```python
from build123d import *

# Parameters (mm, degrees)
F0_W     = 5
F0_H     = 5
F1_DEPTH = 33
F2_R     = 5
F3_DEPTH = 5
F5_DEPTH = 1
F7_W     = 5
F7_H     = 5
F8_DEPTH = 8


with BuildPart() as f1:
    # F0 (on Right) → F1 (new body)
    with BuildSketch(Plane.YZ):
        Rectangle(F0_W, F0_H)
    extrude(amount=F1_DEPTH)

    # F2 (on face) → F3 (join)
    with BuildSketch(Plane.YZ.offset(33)):
        Circle(F2_R)
    extrude(amount=F3_DEPTH)

    # F4 (on face) → F5 (join)
    with BuildSketch(Plane(origin=(0, 0, 0), x_dir=(0, -1, 0), z_dir=(-1, 0, 0))):
        with BuildLine():
            ThreePointArc((0, -2.5), (1.767767, -1.767767), (2.5, 0))
            ThreePointArc((2.5, 0), (1.767767, 1.767767), (0, 2.5))
            ThreePointArc((0, 2.5), (-1.767767, 1.767767), (-2.5, 0))
            ThreePointArc((-2.5, 0), (-1.767767, -1.767767), (0, -2.5))
        make_face()
    extrude(amount=F5_DEPTH)

    # F7 (on face) → F8 (join)
    with BuildSketch(Plane(origin=(-1, 0, 0), x_dir=(0, -1, 0), z_dir=(-1, 0, 0))):
        with Locations((-0.012615, 0.104109)):
            Rectangle(F7_W, F7_H)
    extrude(amount=F8_DEPTH)


solid = f1.part
```
The model under review builds one solid part; all positions refer to its coordinate system, in mm. A direction names the side the tool comes from. Coordinates: 2 decimals unless noted, no trailing zeros. Order: outer loops, then holes, each group sorted by start corner. A loop starts at its lowest first (then second) coordinate and runs counter-clockwise, first axis right, second up. Notation, with made-up numbers: (-1.5, -34.5) -> (51.5, -34.5) arc R17 ccw to (51.5, -8.5) -> close; hole circle Ø1 at (-2.5, -26.75). An arc over 180 degrees is marked (long way). Answer in a Markdown table with one row per item. Add a question column.
Item 1: Mouldability with a two-part tool opening along X and no side actions: class faces 6 (the flat face through (-9, 0, 0)), 7 (the flat face through (-1, 1.32, 2.34)), 8 (the flat face through (16, 0, -2.5)) as +X half, -X half, draft (parallel to the pull), parting line (faces both ways), or undercut.
Item 2: Clearance check with flat-ended pins moving along their axes: pin 1 (6 mm diameter, centred on x = 25.5, y = -3, fed in from +Z); pin 2 (4 mm diameter, centred on x = 12.5, y = 2, fed in from -Z); pin 3 (2.5 mm diameter, centred on x = 23, z = -1, fed in from -Y). State where each tip first meets the part, or that it passes through.
Item 3: We need section A-A on z = 1.75. Write out the cut boundary in (x, y), plus the area to 3 significant figures.
Item 4: We need section B-B on x = -6. Write out the cut boundary in (y, z).
Item 5: We need section C-C on y = -4.5. Write out the cut boundary in (x, z), plus the area to 3 significant figures.
Item 6: We need section D-D on z = -2. Write out the cut boundary in (x, y).
Item 7: Machinability: for faces 1 (the flat face through (0, 2, -2)), 2 (the flat face through (-5, -2.487, 0)), 3 (the flat face through (0, 2, 2)), 4 (the flat face through (0, -2, 2)), 5 (the flat face through (-5, 0, 2.604)), which of the approach directions +Z, -Z, +X, -X, +Y, -Y give a long, thin tool a straight path to every point of the face, cutting with its end or side? Answer none if there is none.
Item 8: To check wall thickness, follow probe 1 along X at (y, z) = (3.25, 2.75); probe 2 along Z at (x, y) = (22.5, 1). State the ranges of each line that lie inside material, in increasing order.
Final values:
| question | item | result |
|---|---|---|
| 1 | face 6 | -X half |
| 1 | face 7 | undercut |
| 1 | face 8 | draft |
| 2 | pin 1 | stops at z = 2.5 |
| 2 | pin 2 | stops at z = -2.5 |
| 2 | pin 3 | stops at y = -2.5 |
| 3 | outline | (-9, -2.49) -> (-1, -2.49) -> (-1, -1.79) -> (0, -1.79) -> (0, -2.5) -> (33, -2.5) -> (33, -4.68) -> (38, -4.68) -> (38, 4.68) -> (33, 4.68) -> (33, 2.5) -> (0, 2.5) -> (0, 1.79) -> (-1, 1.79) -> (-1, 2.51) -> (-9, 2.51) -> close |
| 3 | area | 255 mm2 |
| 4 | outline | (-2.49, -2.4) -> (2.51, -2.4) -> (2.51, 2.6) -> (-2.49, 2.6) -> close |
| 5 | outline | (33, -2.18) -> (38, -2.18) -> (38, 2.18) -> (33, 2.18) -> close |
| 5 | area | 21.8 mm2 |
| 6 | outline | (-9, -2.49) -> (-1, -2.49) -> (-1, -1.5) -> (0, -1.5) -> (0, -2.5) -> (33, -2.5) -> (33, -4.58) -> (38, -4.58) -> (38, 4.58) -> (33, 4.58) -> (33, 2.5) -> (0, 2.5) -> (0, 1.5) -> (-1, 1.5) -> (-1, 2.51) -> (-9, 2.51) -> close |
| 7 | face 1 | -Z, +Y |
| 7 | face 2 | +Z, -Z, -X, -Y |
| 7 | face 3 | +Z, +Y |
| 7 | face 4 | +Z, -Y |
| 7 | face 5 | +Z, -X, +Y, -Y |
| 8 | probe 1 | x = 33 to 38 |
| 8 | probe 2 | z = -2.5 to 2.5 |
